Input: part model. Units: mm. Frame: model coordinates. A direction names the side the tool comes from. Give positions to 0.01 mm unless a question says otherwise; leave off trailing zeros. Write each loop counter-clockwise with the first axis right and the second up, starting at its lowest first coordinate (ties: lowest second). Pieces come first, ordered by that corner, then holes. Notation, with made-up numbers: (-39, 55) - (17, 55) arc R15 cw to (17, 74) - close; hole circle Ø4 at (66.5, 88.5). An arc over 180 degrees is marked (long way). Answer as a JSON object with one key per item and string values. Group by question number.
from build123d import *

# Parameters (mm, degrees)
BOSS_EXTRUDE2_DEPTH = 431.8
SKETCH8_R           = 3.175
CUT_EXTRUDE6_DEPTH  = 2.54


with BuildPart() as part:
    # Sketch3 → Boss-Extrude2 (new body)
    with BuildSketch(Plane.XY):
        Polygon((49.2125, 1.5875), (49.2125, 50.8), (50.8, 50.8), (50.8, 1.524), (100.0125, 1.524), (100.0125, 0), (49.2125, 0), align=None)
    extrude(amount=BOSS_EXTRUDE2_DEPTH)

    # Sketch8 → Cut-Extrude6 (cut)
    with BuildSketch(Plane(origin=(50.8, 0, 0), x_dir=(0, 0, -1), z_dir=(1, 0, 0))):
        with Locations((-29.464, 26.416)):
            Circle(SKETCH8_R)
        with BuildLine():
            Line((-245.364, 12.7), (-373.888, 12.7))
            ThreePointArc((-373.888, 12.7), (-388.112, 26.924), (-373.888, 41.148))
            Line((-373.888, 41.148), (-245.364, 41.148))
            ThreePointArc((-245.364, 41.148), (-231.14, 26.924), (-245.364, 12.7))
        make_face()
    extrude(amount=-CUT_EXTRUDE6_DEPTH, mode=Mode.SUBTRACT)


solid = part.part
1) Reachability of faces 4 (the face through (50.017, 27.237, 231.143)), 5 (the face through (50.8, 27, 213)), 6 (the face through (75, 0, 213)) from +Z, -Z, +X, -X, +Y, -Y: full face, straight path, thin tool, end or side. Return the list, or none.
2) Line query: line 1 along Y through (x, z) = (98, 105); line 2 along X through (y, z) = (28.5, 135). Output: solid intervals per line, ascending. Write a range as from..to.
3) Cut plane D-D on y = 37. Return the cut outline in (x, z).
4) Mould query, pull axis Y, two halves, no side actions, for faces 1 (the face through (63, 1, 0)), 2 (the face through (50.02, 26.61, 388.11)), 3 (the face through (75, 1.524, 213)). Classes: +Y half, -Y half, draft (parallel to the pull), parting line (faces both ways), or undercut.
5) Pin query (flat end, axial travel): P1, Ø8, axis at y = 12, z = 243, coming from the +X side; P2, Ø24.5, axis at x = 73, z = 307, coming from the +Y side. Return the tip coordinate at first contact, or that it passes through.
6) Cut plane B-B on y = 18. Return the cut outline in (x, z).
7) Cut plane C-C on z = 80.5. Return the cut outline in (x, y).
8) Cut plane A-A on z = 282.5. Return the cut outline in (x, y).
Filled in:
{
 "1": {"face 4": "+X, -X", "face 5": "+Z, -Z, +X, +Y", "face 6": "+Z, -Z, +X, -X, -Y"},
 "2": {"line 1": "y = 0..1.52", "line 2": "x = 49.21..50.8"},
 "3": {"outline": "(49.21, 0) - (50.8, 0) - (50.8, 235.32) - (49.21, 235.32) - close; (49.21, 383.93) - (50.8, 383.93) - (50.8, 431.8) - (49.21, 431.8) - close"},
 "4": {"face 1": "draft", "face 2": "undercut", "face 3": "+Y half"},
 "5": {"P1": "stops at x = 50.8", "P2": "stops at y = 1.52"},
 "6": {"outline": "(49.21, 0) - (50.8, 0) - (50.8, 234.29) - (49.21, 234.29) - close; (49.21, 384.96) - (50.8, 384.96) - (50.8, 431.8) - (49.21, 431.8) - close"},
 "7": {"outline": "(49.21, 0) - (100.01, 0) - (100.01, 1.52) - (50.8, 1.52) - (50.8, 50.8) - (49.21, 50.8) - close"},
 "8": {"outline": "(49.21, 0) - (100.01, 0) - (100.01, 1.52) - (50.8, 1.52) - (50.8, 12.7) - (49.21, 12.7) - close; (49.21, 41.15) - (50.8, 41.15) - (50.8, 50.8) - (49.21, 50.8) - close"}
}
